Part model, mm, in its own coordinate system. Face numbers are marked on the shaded views. A direction names the side the tool comes from. Give positions to 0.01 mm unless a question says otherwise; leave off trailing zeros. Write each loop counter-clockwise with the first axis right and the second up, starting at its lowest first coordinate (ties: lowest second). Pieces come first, ordered by that corner, then holes. Notation, with made-up numbers: (2, 83.5) - (57, 83.5) arc R15 ccw to (57, 110.5) - close; hole circle Ø7 at (83.25, -31). An arc over 180 degrees is marked (long way). Answer as a JSON object with one key per item and string values. Group by question number.
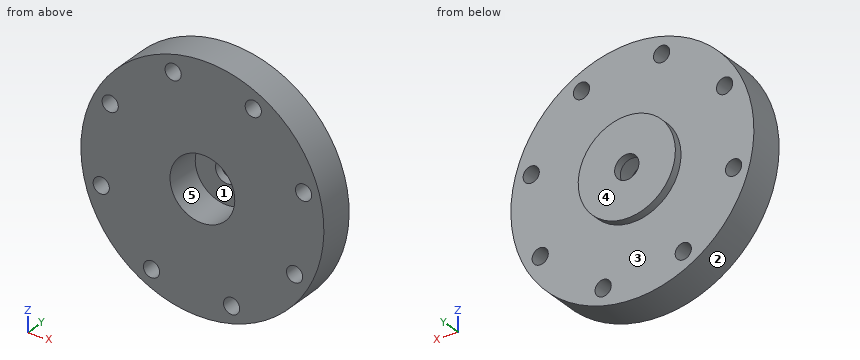
```python
from build123d import *

# Parameters (mm, degrees)
SKETCH_1_R          = 15
EXTRUDE_1_DEPTH     = 2.25
SKETCH_2_R          = 6
EXTRUDE_2_DEPTH     = 1
SKETCH_3_R          = 1
CUT_EXTRUDE_1_DEPTH = 5
SKETCH_4_R          = 4
CUT_EXTRUDE_2_DEPTH = 4.5
SKETCH_5_R          = 1.5
CUT_EXTRUDE_3_DEPTH = 4.5


with BuildPart() as part:
    # ｽｹｯﾁ1 → ﾎﾞｽ - 押し出し1 (new, symmetric)
    with BuildSketch(Plane(origin=(0, 0, 0), x_dir=(1, 0, 0), z_dir=(0, 1, 0))):
        with Locations(Location((0, 0, 0), (0, 0, 270))):
            Circle(SKETCH_1_R)
    extrude(amount=EXTRUDE_1_DEPTH, both=True)

    # ｽｹｯﾁ2 → ﾎﾞｽ - 押し出し2 (add)
    with BuildSketch(Plane(origin=(0, 2.25, 0), x_dir=(1, 0, 0), z_dir=(0, 1, 0))):
        with Locations(Location((0, 0, 0), (0, 0, 270))):
            Circle(SKETCH_2_R)
    extrude(amount=EXTRUDE_2_DEPTH)

    # ｽｹｯﾁ3 → ｶｯﾄ - 押し出し1 (cut)
    with BuildSketch(Plane(origin=(0, 2.25, 0), x_dir=(1, 0, 0), z_dir=(0, 1, 0))):
        with Locations(Location((-11.382561056, -6.279912723, 0), (0, 0, 270))):
            Circle(SKETCH_3_R)
        with Locations(Location((-12.489254982, 3.608117238, 0), (0, 0, 270))):
            Circle(SKETCH_3_R)
        with Locations(Location((-6.279912723, 11.382561056, 0), (0, 0, 270))):
            Circle(SKETCH_3_R)
        with Locations(Location((3.608117238, 12.489254982, 0), (0, 0, 270))):
            Circle(SKETCH_3_R)
        with Locations(Location((11.382561056, 6.279912723, 0), (0, 0, 270))):
            Circle(SKETCH_3_R)
        with Locations(Location((12.489254982, -3.608117238, 0), (0, 0, 270))):
            Circle(SKETCH_3_R)
        with Locations(Location((6.279912723, -11.382561056, 0), (0, 0, 270))):
            Circle(SKETCH_3_R)
        with Locations(Location((-3.608117238, -12.489254982, 0), (0, 0, 270))):
            Circle(SKETCH_3_R)
    extrude(amount=-CUT_EXTRUDE_1_DEPTH, mode=Mode.SUBTRACT)

    # ｽｹｯﾁ4 → ｶｯﾄ - 押し出し2 (cut)
    with BuildSketch(Plane.XZ.offset(2.25)):
        with Locations(Location((0, 0, 0), (0, 0, 270))):
            Circle(SKETCH_4_R)
    extrude(amount=-CUT_EXTRUDE_2_DEPTH, mode=Mode.SUBTRACT)

    # ｽｹｯﾁ5 → ｶｯﾄ - 押し出し3 (cut)
    with BuildSketch(Plane(origin=(0, 3.25, 0), x_dir=(1, 0, 0), z_dir=(0, 1, 0))):
        with Locations(Location((0, 0, 0), (0, 0, 270))):
            Circle(SKETCH_5_R)
    extrude(amount=-CUT_EXTRUDE_3_DEPTH, mode=Mode.SUBTRACT)


solid = part.part
```
1) Saw through at D-D (z = -6.5). List the corners of the cut face in (x, y), and give its area (3 significant figures).
2) Two-plate mould, pull along X, no slides. Class the marked faces 1, 2 and 3: +X half, -X half, draft (parallel to the pull), parting line (faces both ways), or undercut.
3) Saw through at C-C (y = -0.6). State how many separate pieces and enclosed holes the cut face has, and give its area (3 significant figures).
4) Saw through at B-B (z = 0). List the corners of the cut face in (x, y).
5) Saw through at A-A (x = 0). List the corners of the cut face in (y, z).
6) Drill centre lines: line 1 along X through (y, z) = (2.9, 0); line 2 along Y through (x, z) = (12.75, 6); line 3 along Z through (x, y) = (-5.75, -1.2). Where is each one in solid material? Low to high. Write a range as from..to.
7) Which spindle directions (+Z, -Z, +X, -X, +Y, -Y) get a long thin tool onto all of the face, cutting with end or side? Do the marked faces 4 and 5. Say none if no direction does.
8) Drop flat-ended pins along their axis: P1, Ø5, axis at x = -4.5, z = -11.5, coming from the +Y side; P2, Ø1.5, axis at x = 4, y = -1, coming from the +Z side; P3, Ø1.5, axis at x = -1, y = -0.5, coming from the +Z side. Give the stop position or say it passes through.
Checks:
{
 "1": {"outline": "(-13.52, -2.25) - (10.41, -2.25) - (10.41, 2.25) - (-13.52, 2.25) - close; (12.36, -2.25) - (13.52, -2.25) - (13.52, 2.25) - (12.36, 2.25) - close", "area": "113 mm2"},
 "2": {"face 1": "undercut", "face 2": "parting line", "face 3": "draft"},
 "3": {"separate pieces": "1", "enclosed holes": "9", "area": "631 mm2"},
 "4": {"outline": "(-15, -2.25) - (-4, -2.25) - (-4, 2.25) - (-1.5, 2.25) - (-1.5, 3.25) - (-6, 3.25) - (-6, 2.25) - (-15, 2.25) - close; (1.5, 2.25) - (4, 2.25) - (4, -2.25) - (15, -2.25) - (15, 2.25) - (6, 2.25) - (6, 3.25) - (1.5, 3.25) - close"},
 "5": {"outline": "(-2.25, -15) - (2.25, -15) - (2.25, -6) - (3.25, -6) - (3.25, -1.5) - (2.25, -1.5) - (2.25, -4) - (-2.25, -4) - close; (-2.25, 4) - (2.25, 4) - (2.25, 1.5) - (3.25, 1.5) - (3.25, 6) - (2.25, 6) - (2.25, 15) - (-2.25, 15) - close"},
 "6": {"line 1": "-6..-1.5, 1.5..6", "line 2": "-2.25..2.25", "line 3": "-13.85..-12.23, -10.53..13.85"},
 "7": {"face 4": "+Z, -Z, +X, -X, +Y", "face 5": "-Y"},
 "8": {"P1": "y = 2.25", "P2": "z = 14.64", "P3": "z = 15"}
}
